Geometry check sheet. Reference: the model listing, model coordinates, mm. Give positions to 0.01 mm unless a question says otherwise; leave off trailing zeros. Loops run counter-clockwise (first coordinate to the right, second up) from the corner with the lowest first, then second, coordinate; pieces in that order, holes last.
1. Cross-section at A-A, the plane z = 0. Record the cut outline in (x, y), plus the area to 3 significant figures.
2. Cross-section at B-B, the plane y = 22. Record the cut outline in (x, z).
3. Cross-section at C-C, the plane x = 26.5. Record the cut outline in (y, z), plus the area to 3 significant figures.
4. Material ranges on L1, parallel to Y at x = 28.55, z = -5; L2, parallel to Y at x = 27.45, z = 7; L3, parallel to Z at x = 25.55, y = 24, recorded low to high.
from build123d import *

# Parameters (mm, degrees)
SKETCH_1_W          = 34
SKETCH_1_H          = 32
SKETCH_1_R          = 1.5
EXTRUDE_1_DEPTH     = 4
SKETCH_2_W          = 17
SKETCH_2_H          = 4
CUT_EXTRUDE_1_DEPTH = 5


with BuildPart() as part:
    # Эскиз1 → Бобышка-Вытянуть1 (new body)
    with BuildSketch(Plane(origin=(25.2, 0, 0), x_dir=(0, 0, -1), z_dir=(1, 0, 0))):
        with Locations((3.763696673, 23.493617857)):
            Rectangle(SKETCH_1_W, SKETCH_1_H)
        with Locations((-6.236303327, 31.493617857)):
            Circle(SKETCH_1_R, mode=Mode.SUBTRACT)
        with Locations((13.763696673, 31.493617857)):
            Circle(SKETCH_1_R, mode=Mode.SUBTRACT)
        with Locations((-6.236303327, 15.493617857)):
            Circle(SKETCH_1_R, mode=Mode.SUBTRACT)
        with Locations((13.763696673, 15.493617857)):
            Circle(SKETCH_1_R, mode=Mode.SUBTRACT)
    extrude(amount=EXTRUDE_1_DEPTH)

    # Эскиз2 → Вырез-Вытянуть1 (cut, through all)
    with BuildSketch(Plane(origin=(29.2, 0, 0), x_dir=(0, 0, -1), z_dir=(1, 0, 0))):
        with Locations((3.763696673, 23.493617857)):
            Rectangle(SKETCH_2_W, SKETCH_2_H)
    extrude(amount=-CUT_EXTRUDE_1_DEPTH, mode=Mode.SUBTRACT)


solid = part.part
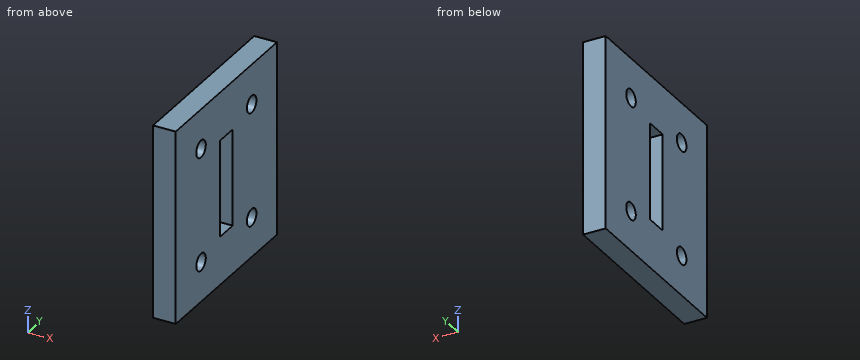
Result:
1. outline: (25.2, 7.49) - (29.2, 7.49) - (29.2, 21.49) - (25.2, 21.49) - close; (25.2, 25.49) - (29.2, 25.49) - (29.2, 39.49) - (25.2, 39.49) - close
1. area: 112 mm2
2. outline: (25.2, -20.76) - (29.2, -20.76) - (29.2, -12.26) - (25.2, -12.26) - close; (25.2, 4.74) - (29.2, 4.74) - (29.2, 13.24) - (25.2, 13.24) - close
3. outline: (7.49, -20.76) - (39.49, -20.76) - (39.49, 13.24) - (7.49, 13.24) - close; hole circle Ø3 at (15.49, -13.76); hole circle Ø3 at (15.49, 6.24); hole (21.49, -12.26) - (25.49, -12.26) - (25.49, 4.74) - (21.49, 4.74) - close; hole circle Ø3 at (31.49, -13.76); hole circle Ø3 at (31.49, 6.24)
3. area: 992 mm2
4. L1: y = 7.49 to 21.49, 25.49 to 39.49
4. L2: y = 7.49 to 14.2, 16.78 to 30.2, 32.78 to 39.49
4. L3: z = -20.76 to -12.26, 4.74 to 13.24
